```python
from build123d import *

# Parameters (mm, degrees)
SKETCH1_W           = 228.6
SKETCH1_H           = 76.2
SKETCH1_R           = 3.048
SKETCH1_R_2         = 5.08
BOSS_EXTRUDE1_DEPTH = 3.175
SKETCH2_W           = 12.7
SKETCH2_H           = 3.175
BOSS_EXTRUDE2_DEPTH = 3.175
SKETCH3_W           = 22.86
SKETCH3_H           = 25.4
CUT_EXTRUDE1_DEPTH  = 4.175
SKETCH4_W           = 3.175
SKETCH4_H           = 12.7
BOSS_EXTRUDE3_DEPTH = 3.175
SKETCH6_R           = 2.25
CUT_EXTRUDE2_DEPTH  = 4.175
SKETCH8_W           = 10.16
SKETCH8_H           = 50.8
CUT_EXTRUDE3_DEPTH  = 4.175
SKETCH12_W          = 3.175
SKETCH12_H          = 6.35
CUT_EXTRUDE5_DEPTH  = 3.175
CUT_EXTRUDE6_DEPTH  = 4.175
SKETCH14_W          = 6.35
SKETCH14_H          = 3.175
CUT_EXTRUDE7_DEPTH  = 4.175
CUT_EXTRUDE8_DEPTH  = 4.175
CUT_EXTRUDE9_DEPTH  = 4.175


with BuildPart() as part:
    # Sketch1 → Boss-Extrude1 (new body)
    with BuildSketch(Plane.XY):
        with Locations((114.3, 38.1)):
            Rectangle(SKETCH1_W, SKETCH1_H)
        with Locations((215.9, 30.48)):
            Circle(SKETCH1_R, mode=Mode.SUBTRACT)
        with Locations((92.075, 30.48)):
            Circle(SKETCH1_R, mode=Mode.SUBTRACT)
        with Locations((41.56075, 30.48)):
            Circle(SKETCH1_R_2, mode=Mode.SUBTRACT)
    extrude(amount=BOSS_EXTRUDE1_DEPTH)

    # Sketch2 → Boss-Extrude2 (add)
    with BuildSketch(Plane.XZ):
        with Locations((222.25, 1.5875)):
            Rectangle(SKETCH2_W, SKETCH2_H)
        with Locations((196.85, 1.5875)):
            Rectangle(SKETCH2_W, SKETCH2_H)
        with Locations((171.45, 1.5875)):
            Rectangle(SKETCH2_W, SKETCH2_H)
        with Locations((146.05, 1.5875)):
            Rectangle(SKETCH2_W, SKETCH2_H)
        with Locations((120.65, 1.5875)):
            Rectangle(SKETCH2_W, SKETCH2_H)
        with Locations((95.25, 1.5875)):
            Rectangle(SKETCH2_W, SKETCH2_H)
        with Locations((69.85, 1.5875)):
            Rectangle(SKETCH2_W, SKETCH2_H)
        with Locations((44.45, 1.5875)):
            Rectangle(SKETCH2_W, SKETCH2_H)
    extrude(amount=BOSS_EXTRUDE2_DEPTH)

    # Sketch3 → Cut-Extrude1 (cut, through all)
    with BuildSketch(Plane(origin=(0, 0, 0), x_dir=(-1, 0, 0), z_dir=(0, 0, -1))):
        with Locations((-11.43, 12.7)):
            Rectangle(SKETCH3_W, SKETCH3_H)
    extrude(amount=-CUT_EXTRUDE1_DEPTH, mode=Mode.SUBTRACT)

    # Sketch4 → Boss-Extrude3 (add)
    with BuildSketch(Plane.ZY.offset(-22.86)):
        with Locations((1.5875, 6.35)):
            Rectangle(SKETCH4_W, SKETCH4_H)
    extrude(amount=BOSS_EXTRUDE3_DEPTH)

    # Sketch6 → Cut-Extrude2 (cut, through all)
    with BuildSketch(Plane(origin=(0, 0, 0), x_dir=(-1, 0, 0), z_dir=(0, 0, -1))):
        with Locations((-27.16075, 35.48)):
            Circle(SKETCH6_R)
        with Locations((-27.16075, 25.48)):
            Circle(SKETCH6_R)
        with Locations((-76.66075, 35.48)):
            Circle(SKETCH6_R)
        with Locations((-76.66075, 25.48)):
            Circle(SKETCH6_R)
    extrude(amount=-CUT_EXTRUDE2_DEPTH, mode=Mode.SUBTRACT)

    # Sketch8 → Cut-Extrude3 (cut, through all)
    with BuildSketch(Plane.XY.offset(3.175)):
        with Locations((5.08, 50.8)):
            Rectangle(SKETCH8_W, SKETCH8_H)
    extrude(amount=-CUT_EXTRUDE3_DEPTH, mode=Mode.SUBTRACT)

    # Sketch12 → Cut-Extrude5 (cut)
    with BuildSketch(Plane(origin=(0, 0, 0), x_dir=(-1, 0, 0), z_dir=(0, 0, -1))):
        with Locations((-220.6625, 66.675)):
            Rectangle(SKETCH12_W, SKETCH12_H)
        with Locations((-174.9425, 66.675)):
            Rectangle(SKETCH12_W, SKETCH12_H)
        with Locations((-129.2225, 66.675)):
            Rectangle(SKETCH12_W, SKETCH12_H)
        with Locations((-83.5025, 66.675)):
            Rectangle(SKETCH12_W, SKETCH12_H)
        with Locations((-37.7825, 66.675)):
            Rectangle(SKETCH12_W, SKETCH12_H)
    extrude(amount=-CUT_EXTRUDE5_DEPTH, mode=Mode.SUBTRACT)

    # Sketch13 → Cut-Extrude6 (cut, through all)
    with BuildSketch(Plane.XY.offset(3.175)):
        with BuildLine():
            Line((10.16, 60.96), (10.16, 76.2))
            Line((10.16, 76.2), (25.4, 76.2))
            ThreePointArc((25.4, 76.2), (14.623692655, 71.736307345), (10.16, 60.96))
        make_face()
    extrude(amount=-CUT_EXTRUDE6_DEPTH, mode=Mode.SUBTRACT)

    # Sketch14 → Cut-Extrude7 (cut, through all)
    with BuildSketch(Plane.XY.offset(3.175)):
        with Locations((17.145, 32.0675)):
            Rectangle(SKETCH14_W, SKETCH14_H)
        with Locations((17.145, 47.3075)):
            Rectangle(SKETCH14_W, SKETCH14_H)
    extrude(amount=-CUT_EXTRUDE7_DEPTH, mode=Mode.SUBTRACT)

    # Sketch15 → Cut-Extrude8 (cut, through all)
    with BuildSketch(Plane.XY.offset(3.175)):
        Polygon((26.639339978, 64.870175511), (26.085901012, 71.196011844), (29.248819178, 71.472731328), (29.802258145, 65.146894995), align=None)
    extrude(amount=-CUT_EXTRUDE8_DEPTH, mode=Mode.SUBTRACT)

    # Sketch16 → Cut-Extrude9 (cut, through all)
    with BuildSketch(Plane.XY.offset(3.175)):
        with BuildLine():
            Line((218.44, 76.2), (228.6, 76.2))
            Line((228.6, 76.2), (228.6, 66.04))
            ThreePointArc((228.6, 66.04), (225.624204897, 73.224204897), (218.44, 76.2))
        make_face()
    extrude(amount=-CUT_EXTRUDE9_DEPTH, mode=Mode.SUBTRACT)


solid = part.part
```
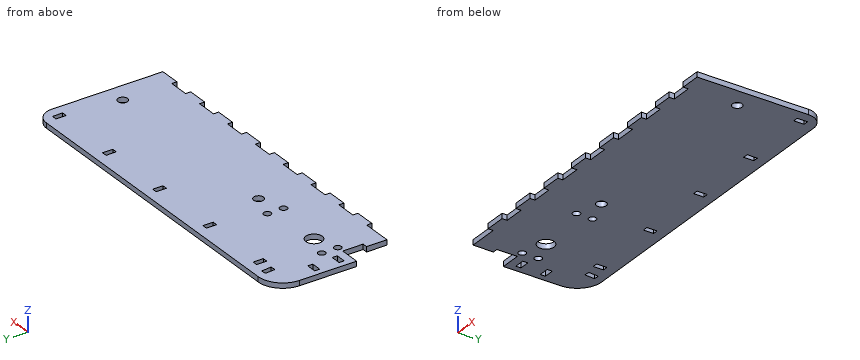
Geometry check sheet. Reference: the model listing, model coordinates, mm. Give positions to 0.01 mm unless a question says otherwise; leave off trailing zeros. Write item = value, one per line. Start each with the question number.
1. Thickness scan on probe 1 along X at (y, z) = (46.5, 1.55); probe 2 along Y at (x, z) = (27, 0.2); probe 3 along X at (y, z) = (34, 2.5). Record the ranges inside material, lowest first.
2. Section check A-A, the plane z = 0.8. Give the number of separate pieces and of enclosed holes in the cut face, plus the area to 3 significant figures.
3. Go/stop test with flat-tipped pins: P1, Ø1.6, axis at y = -1, z = 2.5, coming from the -X side; P2, Ø1, axis at y = 65, z = 1.5, coming from the -X side; P3, Ø1.5, axis at x = 77.5, z = 2.5, coming from the -Y side. Record where each tip stops, or that it passes through.
Values follow:
q1.probe_1 = 10.16 to 13.97, 20.32 to 228.6
q1.probe_2 = 0 to 23.24, 27.72 to 33.24, 37.72 to 64.9, 71.28 to 76.2
q1.probe_3 = 10.16 to 25.47, 28.86 to 37.9, 45.22 to 74.97, 78.36 to 228.6
q2.separate_pieces = 1
q2.enclosed_holes = 15
q2.area = 16,200 mm^2
q3.P1 = 38.1
q3.P2 = 10.58
q3.P3 = 0
